from build123d import *

# Parameters (mm, degrees)
F0_W      = 24
F0_H      = 24
F1_DEPTH  = 20
F3_R      = 24
F3_R_2    = 15
F4_DEPTH  = 24
F6_DEPTH  = 24
F2_R      = 15
F7_DEPTH  = 24
F8_W      = 14
F8_H      = 16
F9_DEPTH  = 65
F10_R     = 9
F11_DEPTH = 35


with BuildPart() as f1:
    # F0 (on Front) → F1 (new body)
    with BuildSketch(Plane.XZ):
        with Locations((12, 12)):
            Rectangle(F0_W, F0_H)
    extrude(amount=-F1_DEPTH)

    # F3 (on face) → F4 (join)
    with BuildSketch(Plane.YZ):
        with Locations((35, 12)):
            Circle(F3_R)
        with Locations((35.131581, 12)):
            Circle(F3_R_2, mode=Mode.SUBTRACT)
    extrude(amount=F4_DEPTH)

    # F5 (on Right) → F6 (join)
    with BuildSketch(Plane.YZ):
        Polygon((35, 31), (35, 0), (35, -7), (100, -7), (100, 31), align=None)
    extrude(amount=F6_DEPTH)

    # F2 (on Right) → F7 (cut)
    with BuildSketch(Plane.YZ):
        with Locations((35.131581, 12)):
            Circle(F2_R)
    extrude(amount=F7_DEPTH, mode=Mode.SUBTRACT)

    # F8 (on face) → F9 (cut)
    with BuildSketch(Plane(origin=(0, 100, 0), x_dir=(-1, 0, 0), z_dir=(0, 1, 0))):
        with Locations((-17, 12)):
            Rectangle(F8_W, F8_H)
    extrude(amount=-F9_DEPTH, mode=Mode.SUBTRACT)

    # F10 (on face) → F11 (cut)
    with BuildSketch(Plane.XZ):
        with Locations((12, 12)):
            Circle(F10_R)
    extrude(amount=-F11_DEPTH, mode=Mode.SUBTRACT)


solid = f1.part
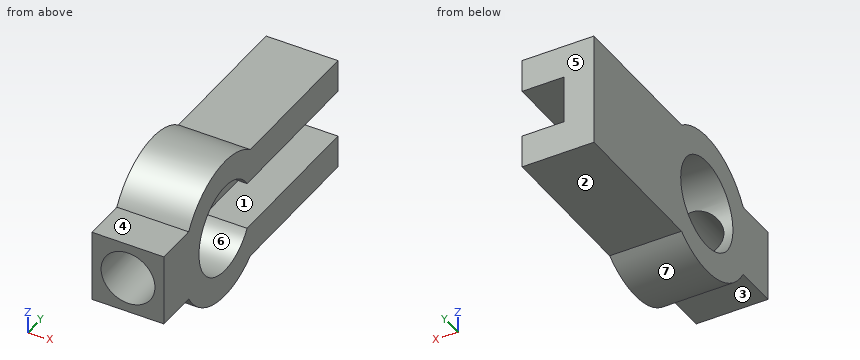
The model under review builds one solid part; all positions refer to its coordinate system, in mm. Face numbers are marked on the shaded views. A direction names the side the tool comes from. Give positions to 0.01 mm unless a question says otherwise; leave off trailing zeros. Order: outer loops, then holes, each group sorted by start corner. A loop starts at its lowest first (then second) coordinate and runs counter-clockwise, first axis right, second up. Notation, with made-up numbers: (9, 61.25) -> (60, 61.25) arc R14 ccw to (60, 82.25) -> close; hole circle Ø2 at (59.25, 18.5). An arc over 180 degrees is marked (long way). Write item = value, one per line. Start each with the question number.
(1) Tool access review of the marked faces 1, 2, 3 and 4: name each direction out of +Z, -Z, +X, -X, +Y, -Y from which nothing blocks a thin tool from reaching the whole face with its end or side.
(2) Take a section at C-C (y = 60.5). Write out the cut boundary in (x, z).
(3) Take a section at A-A (z = 12). Write out the cut boundary in (x, y), plus the area to 3 significant figures.
(4) Take a section at B-B (x = 12). Write out the cut boundary in (y, z), plus the area to 3 significant figures.
(5) For pin 1 Ø7 at (x, y) = (17.5, 70) entering from +Z; pin 2 Ø3 at (x, z) = (11.5, -5.5) entering from -Y; pin 3 Ø11 at (x, y) = (18.5, 86.5) entering from -Z; pin 4 Ø18 at (y, z) = (35.13, 12) entering from +X, all flat-tipped, find the tip position at first contact; note any pin that passes through.
(6) Take a section at D-D (z = 23). Write out the cut boundary in (x, y), plus the area to 3 significant figures.
(7) Draft analysis for pull direction Y (two halves, no side actions). For the marked faces 5, 6 and 7, state which applies: +Y half, -Y half, draft (parallel to the pull), parting line (faces both ways), or undercut.
(8) For L1, parallel to Z at x = 21.5, y = 85; L2, parallel to X at y = 8, z = 12, list the stretches that pass through material, from the lowest coordinate up. Write a range as from..to.
Returned:
q1.face_1 = +X, +Y
q1.face_2 = -Z, +X, -X, +Y
q1.face_3 = -Z, +X, -X, -Y
q1.face_4 = +Z, +X, -X, -Y
q2.outline = (0, -7) -> (24, -7) -> (24, 4) -> (10, 4) -> (10, 20) -> (24, 20) -> (24, 31) -> (0, 31) -> close
q3.outline = (0, 0) -> (3, 0) -> (3, 20.13) -> (0, 20.13) -> close; (0, 50.13) -> (10, 50.13) -> (10, 100) -> (0, 100) -> close; (21, 0) -> (24, 0) -> (24, 20.13) -> (21, 20.13) -> close
q3.area = 619 mm²
q4.outline = (0, 0) -> (14.22, 0) arc R24 ccw to (49.66, -7) -> (100, -7) -> (100, 4) -> (47.82, 4) arc R15 cw to (23.13, 3) -> (0, 3) -> close; (0, 21) -> (23.13, 21) arc R15 cw to (47.82, 20) -> (100, 20) -> (100, 31) -> (49.66, 31) arc R24 ccw to (14.22, 24) -> (0, 24) -> close
q4.area = 1,870 mm²
q5.pin_1 = 31
q5.pin_2 = 17.11
q5.pin_3 = -7
q5.pin_4 = through
q6.outline = (0, 0) -> (24, 0) -> (24, 24.93) -> (0, 24.93) -> close; (0, 45.33) -> (24, 45.33) -> (24, 100) -> (0, 100) -> close
q6.area = 1,910 mm²
q7.face_5 = +Y half
q7.face_6 = undercut
q7.face_7 = parting line
q8.L1 = -7..4, 20..31
q8.L2 = 0..3, 21..24
